```python
from build123d import *

# Parameters (mm, degrees)
SKETCH1_R           = 3
SKETCH1_R_2         = 2.15
BOSS_EXTRUDE1_DEPTH = 10
FILLET1_R           = 0.35


with BuildPart() as part:
    # Sketch1 → Boss-Extrude1 (new body)
    # profile 1 of 10: a face of its own
    with BuildSketch(Plane(origin=(0, 0, 0), x_dir=(1, 0, 0), z_dir=(0, 1, 0))):
        with BuildLine():
            Line((1, 2.828427125), (0, 4.25))
            Line((0, 4.25), (-1, 2.828427125))
            ThreePointArc((-1, 2.828427125), (0, 3), (1, 2.828427125))
        make_face()
    # profile 2 of 10: a face of its own
    with BuildSketch(Plane(origin=(0, 0, 0), x_dir=(1, 0, 0), z_dir=(0, 1, 0))):
        with BuildLine():
            Line((2.731847341, 3.255688883), (1.052033468, 2.809488491))
            ThreePointArc((1.052033468, 2.809488491), (1.928362829, 2.298133329), (2.584122354, 1.523913272))
            Line((2.584122354, 1.523913272), (2.731847341, 3.255688883))
        make_face()
    # profile 3 of 10: a face of its own
    with BuildSketch(Plane(origin=(0, 0, 0), x_dir=(1, 0, 0), z_dir=(0, 1, 0))):
        with BuildLine():
            Line((4.18543295, 0.738004755), (2.611808784, 1.475958969))
            ThreePointArc((2.611808784, 1.475958969), (2.901329553, 0.763077207), (3, 0))
            ThreePointArc((3, 0), (2.989758804, -0.24767376), (2.959105139, -0.493656537))
            Line((2.959105139, -0.493656537), (4.18543295, 0.738004755))
        make_face()
    # profile 4 of 10: a face of its own
    with BuildSketch(Plane(origin=(0, 0, 0), x_dir=(1, 0, 0), z_dir=(0, 1, 0))):
        with BuildLine():
            Line((3.680607966, -2.125), (2.949489743, -0.548188159))
            ThreePointArc((2.949489743, -0.548188159), (2.598076211, -1.5), (1.949489743, -2.280238966))
            Line((1.949489743, -2.280238966), (3.680607966, -2.125))
        make_face()
    # profile 5 of 10: a face of its own
    with BuildSketch(Plane(origin=(0, 0, 0), x_dir=(1, 0, 0), z_dir=(0, 1, 0))):
        with BuildLine():
            Line((1.453585609, -3.993693638), (1.907071671, -2.315831954))
            ThreePointArc((1.907071671, -2.315831954), (1.02606043, -2.819077862), (0.02768643, -2.999872241))
            Line((0.02768643, -2.999872241), (1.453585609, -3.993693638))
        make_face()
    # profile 6 of 10: a face of its own
    with BuildSketch(Plane(origin=(0, 0, 0), x_dir=(1, 0, 0), z_dir=(0, 1, 0))):
        with BuildLine():
            ThreePointArc((-0.02768643, -2.999872241), (-1.02606043, -2.819077862), (-1.907071671, -2.315831954))
            Line((-1.907071671, -2.315831954), (-1.453585609, -3.993693638))
            Line((-1.453585609, -3.993693638), (-0.02768643, -2.999872241))
        make_face()
    # profile 7 of 10: a face of its own
    with BuildSketch(Plane(origin=(0, 0, 0), x_dir=(1, 0, 0), z_dir=(0, 1, 0))):
        Circle(SKETCH1_R)
        with Locations(Location((0, 0, 0), (0, 0, 270))):
            Circle(SKETCH1_R_2, mode=Mode.SUBTRACT)
    # profile 8 of 10: a face of its own
    with BuildSketch(Plane(origin=(0, 0, 0), x_dir=(1, 0, 0), z_dir=(0, 1, 0))):
        with BuildLine():
            ThreePointArc((-1.949489743, -2.280238966), (-2.598076211, -1.5), (-2.949489743, -0.548188159))
            Line((-2.949489743, -0.548188159), (-3.680607966, -2.125))
            Line((-3.680607966, -2.125), (-1.949489743, -2.280238966))
        make_face()
    # profile 9 of 10: a face of its own
    with BuildSketch(Plane(origin=(0, 0, 0), x_dir=(1, 0, 0), z_dir=(0, 1, 0))):
        with BuildLine():
            ThreePointArc((-2.959105139, -0.493656537), (-2.954423259, 0.520944533), (-2.611808784, 1.475958969))
            Line((-2.611808784, 1.475958969), (-4.18543295, 0.738004755))
            Line((-4.18543295, 0.738004755), (-2.959105139, -0.493656537))
        make_face()
    # profile 10 of 10: a face of its own
    with BuildSketch(Plane(origin=(0, 0, 0), x_dir=(1, 0, 0), z_dir=(0, 1, 0))):
        with BuildLine():
            ThreePointArc((-2.584122354, 1.523913272), (-1.928362829, 2.298133329), (-1.052033468, 2.809488491))
            Line((-1.052033468, 2.809488491), (-2.731847341, 3.255688883))
            Line((-2.731847341, 3.255688883), (-2.584122354, 1.523913272))
        make_face()
    extrude(amount=BOSS_EXTRUDE1_DEPTH)

    # Fillet1
    fillet1_edges = [part.edges().sort_by_distance(p)[0] for p in [
        (0, 5, -4.25),
        (2.731847341, 5, -3.255688883),
        (4.18543295, 5, -0.738004755),
        (3.680607966, 5, 2.125),
        (1.453585609, 5, 3.993693638),
        (-1.453585609, 5, 3.993693638),
        (-3.680607966, 5, 2.125),
        (-4.18543295, 5, -0.738004755),
        (-2.731847341, 5, -3.255688883),
    ]]
    fillet(fillet1_edges, radius=FILLET1_R)


solid = part.part
```
Input: part model. Units: mm. Frame: model coordinates. A direction names the side the tool comes from. Coordinates: 2 decimals unless noted, no trailing zeros. Write each loop counter-clockwise with the first axis right and the second up, starting at its lowest first coordinate (ties: lowest second). Pieces come first, ordered by that corner, then holes. Notation, with made-up numbers: (60, 8.5) -> (96, 8.5) arc R28 ccw to (96, 27.5) -> close; hole circle Ø2 at (-39, 0). An arc over 180 degrees is marked (long way). Write each question's results on one line, items separated by ' | '.
Item 1: Pin query (flat end, axial travel): pin 1 Ø2 at (x, z) = (3, 0.5) entering from +Y; pin 2 Ø3.5 at (x, z) = (0, 0) entering from +Y; pin 3 Ø3 at (x, y) = (2.5, 2) entering from -Z. Return the tip coordinate at first contact, or that it passes through.
Conclusion:
pin 1: stops at y = 10 | pin 2: passes through | pin 3: stops at z = -3.14
Item 2: Section query B-B on z = -3. Return loops of the section in (x, y), plus the area to 3 significant figures.
Conclusion:
outline: (-2.62, 0) -> (-1.77, 0) -> (-1.77, 10) -> (-2.62, 10) -> close; (-0.88, 0) -> (0.88, 0) -> (0.88, 10) -> (-0.88, 10) -> close; (1.77, 0) -> (2.62, 0) -> (2.62, 10) -> (1.77, 10) -> close | area: 34.6 mm^2
Item 3: Section query C-C on x = 0.5. Return loops of the section in (y, z), plus the area to 3 significant figures.
Conclusion:
outline: (0, -3.54) -> (10, -3.54) -> (10, -2.09) -> (0, -2.09) -> close; (0, 2.09) -> (10, 2.09) -> (10, 3.33) -> (0, 3.33) -> close | area: 26.9 mm^2
Item 4: Section query A-A on z = 1. Return loops of the section in (x, y), plus the area to 3 significant figures.
Conclusion:
outline: (-3.16, 0) -> (-1.9, 0) -> (-1.9, 10) -> (-3.16, 10) -> close; (1.9, 0) -> (3.16, 0) -> (3.16, 10) -> (1.9, 10) -> close | area: 25.1 mm^2
Item 5: Mould query, pull axis X, two halves, no side actions, for faces 1 (the flat face through (-2.576, 4.93, 2.224)), 2 (the flat face through (1.66, 4.93, -2.97)), 3 (the flat face through (1.743, 4.93, 2.923)), 4 (the cylindrical face through (-1.308, 4.93, -1.706)). Classes: +X half, -X half, draft (parallel to the pull), parting line (faces both ways), or undercut.
Conclusion:
face 1: -X half | face 2: undercut | face 3: +X half | face 4: undercut
Item 6: Set-up query: faces 5 (the flat face through (-0.64, 4.93, -3.34)), 6 (the flat face through (-0.544, 4.93, 3.359)), 7 (the flat face through (-2.638, 4.93, -2.151)), 8 (the flat face through (2.636, 4.93, -2.133)). Return all of +Z, -Z, +X, -X, +Y, -Y with unobstructed straight access to the full face (end or side cutting, diameter ignored); none if empty.
Conclusion:
face 5: -Z, +Y, -Y | face 6: +Z, +Y, -Y | face 7: -X, +Y, -Y | face 8: +X, +Y, -Y
Item 7: Material intervals for probe 1 along X at (y, z) = (8, 0.25); probe 2 along Z at (x, y) = (3, 6.5); probe 3 along X at (y, z) = (6.5, 0), sorted ascending.
Conclusion:
probe 1: x = -3.2 to -2.14, 2.14 to 3.2 | probe 2: z = -1.29 to 0.45, 0.66 to 2.19 | probe 3: x = -3.45 to -2.15, 2.15 to 3.45
